Verification items for the finished model (mm, model axes). A direction names the side the tool comes from. Coordinates: 2 decimals unless noted, no trailing zeros. Write each loop counter-clockwise with the first axis right and the second up, starting at its lowest first coordinate (ties: lowest second). Pieces come first, ordered by that corner, then holes. Notation, with made-up numbers: (-5.5, 57.25) -> (45.5, 57.25) arc R33 ccw to (45.5, 87.25) -> close; hole circle Ø2 at (8.25, 37). An arc over 180 degrees is marked (long way). Answer in a Markdown table with one row per item.
```python
from build123d import *

# Parameters (mm, degrees)
F0_W      = 82.55
F0_H      = 38.1
F1_DEPTH  = 38.1
F2_W      = 57.15
F2_H      = 25.4
F3_DEPTH  = 38.101
F4_R      = 6.3636745149
F5_DEPTH  = 38.101
F7_DEPTH  = 25.4
F9_DEPTH  = 25.4
F10_DEPTH = 63.501
F12_DEPTH = 25.4


with BuildPart() as f1:
    # F0 (on Front) → F1 (new body)
    with BuildSketch(Plane.XZ):
        with Locations((-41.275, 19.05)):
            Rectangle(F0_W, F0_H)
    extrude(amount=F1_DEPTH)

    # F2 (on face) → F3 (cut, through all)
    with BuildSketch(Plane.XZ.offset(38.1)):
        with Locations((-28.575, 25.4)):
            Rectangle(F2_W, F2_H)
    extrude(amount=-F3_DEPTH, mode=Mode.SUBTRACT)

    # F4 (on face) → F5 (cut, through all)
    with BuildSketch(Plane.XZ.offset(38.1)):
        with Locations((-69.85, 25.9895079914)):
            Circle(F4_R)
    extrude(amount=-F5_DEPTH, mode=Mode.SUBTRACT)

    # F6 (on face) → F7 (cut)
    with BuildSketch(Plane.XY.offset(12.7)):
        with BuildLine():
            ThreePointArc((-43.1306947993, -12.7), (-38.6405667387, -14.5598719395), (-36.7806947993, -19.05))
            ThreePointArc((-36.7806947993, -19.05), (-38.6405667387, -23.5401280605), (-43.1306947993, -25.4))
            Line((-43.1306947993, -25.4), (-17.7306947993, -25.4))
            ThreePointArc((-17.7306947993, -25.4), (-24.0806947993, -19.05), (-17.7306947993, -12.7))
            Line((-17.7306947993, -12.7), (-43.1306947993, -12.7))
        make_face()
        with BuildLine():
            ThreePointArc((-43.1306947993, -25.4), (-38.6405667387, -23.5401280605), (-36.7806947993, -19.05))
            ThreePointArc((-36.7806947993, -19.05), (-38.6405667387, -14.5598719395), (-43.1306947993, -12.7))
            ThreePointArc((-43.1306947993, -12.7), (-49.4806947993, -19.05), (-43.1306947993, -25.4))
        make_face()
        with BuildLine():
            ThreePointArc((-11.3806947993, -19.05), (-13.2405667387, -14.5598719395), (-17.7306947993, -12.7))
            ThreePointArc((-17.7306947993, -12.7), (-24.0806947993, -19.05), (-17.7306947993, -25.4))
            ThreePointArc((-17.7306947993, -25.4), (-13.2405667387, -23.5401280605), (-11.3806947993, -19.05))
        make_face()
    extrude(amount=-F7_DEPTH, mode=Mode.SUBTRACT)

    # F8 (on face) → F9 (join)
    with BuildSketch(Plane.XZ.offset(38.1)):
        with BuildLine():
            ThreePointArc((-67.3090244137, 38.1), (-60.0909334069, 33.7845859546), (-57.15, 25.9058457722))
            Line((-57.15, 25.9058457722), (-57.15, 38.1))
            Line((-57.15, 38.1), (-67.3090244137, 38.1))
        make_face()
        with BuildLine():
            ThreePointArc((-82.55, 26.0334052145), (-79.5712875843, 33.8335010618), (-72.3941565633, 38.1))
            Line((-72.3941565633, 38.1), (-82.55, 38.1))
            Line((-82.55, 38.1), (-82.55, 26.0334052145))
        make_face()
    extrude(amount=F9_DEPTH)

    # F10 (cut, through all): faces of the model
    f10_faces = [f1.faces().sort_by_distance(p)[0] for p in [
        (-59.7492259595, -63.5, 35.2812720031),
        (-79.9507979007, -63.5, 35.2852151474),
    ]]
    extrude(f10_faces, amount=-F10_DEPTH, mode=Mode.SUBTRACT)

    # F11 (on face) → F12 (cut)
    with BuildSketch(Plane.XY.offset(12.7)):
        with BuildLine():
            ThreePointArc((-18.9558640122, 0), (-6.26601343, -5.5476288842), (0, -17.8985628462))
            Line((0, -17.8985628462), (0, 0))
            Line((0, 0), (-18.9558640122, 0))
        make_face()
        with BuildLine():
            ThreePointArc((0, -23.0064517831), (-3.2034542821, -31.7030229504), (-9.9095078185, -38.1))
            Line((-9.9095078185, -38.1), (0, -38.1))
            Line((0, -38.1), (0, -23.0064517831))
        make_face()
    extrude(amount=-F12_DEPTH, mode=Mode.SUBTRACT)


solid = f1.part
```
1. Section check C-C, the plane z = 7. Record the boundary of the cut face in (x, y), plus the area to 3 significant figures.
Geometry says:
| item | result |
|---|---|
| outline | (-82.55, -38.1) -> (-9.91, -38.1) arc R20.5 ccw to (0, -23.01) -> (0, -17.9) arc R20.5 ccw to (-18.96, 0) -> (-82.55, 0) -> close; hole (-43.13, -25.4) -> (-17.73, -25.4) arc R6.35 ccw to (-17.73, -12.7) -> (-43.13, -12.7) arc R6.35 ccw to start |
| area | 2,560 mm^2 |
2. Section check D-D, the plane y = -4.5. Record the boundary of the cut face in (x, z).
Geometry says:
| item | result |
|---|---|
| outline | (-82.55, 0) -> (-7.47, 0) -> (-7.47, 12.7) -> (-57.15, 12.7) -> (-57.15, 25.91) arc R12.7 ccw to (-67.31, 38.1) -> (-72.39, 38.1) arc R12.7 ccw to (-82.55, 26.03) -> close; hole circle Ø12.73 at (-69.85, 25.99) |
3. Tool access check on faces 4 (the flat face through (-30, -12.7, 6)), 5 (the cylindrical face through (-3.13, -31.59, 6.44)), 6 (the flat face through (-29, -28, 12.7)). Record the directions out of +Z, -Z, +X, -X, +Y, -Y that give a thin tool (end or side, any length) a straight path to the whole face; none if there is none.
Geometry says:
| item | result |
|---|---|
| face 4 | +Z, -Z |
| face 5 | +Z, -Z, +X, -Y |
| face 6 | +Z, +X, +Y, -Y |
4. Section check B-B, the plane x = -69.85. Record the boundary of the cut face in (y, z), plus the area to 3 significant figures.
Geometry says:
| item | result |
|---|---|
| outline | (-38.1, 0) -> (0, 0) -> (0, 19.63) -> (-38.1, 19.63) -> close; (-38.1, 32.35) -> (0, 32.35) -> (0, 38.1) -> (-38.1, 38.1) -> close |
| area | 967 mm^2 |
5. Mould release check, pull along Y, two halves, no side actions. Record for faces 1 (the cylindrical face through (-60.17, -19.32, 33.88)), 2 (the cylindrical face through (-49.48, -18.91, 6.44)), 3 (the flat face through (-58, 0, 15)): released by +Y, released by -Y, zero draft, split by the parting line, or undercut.
Geometry says:
| item | result |
|---|---|
| face 1 | zero draft |
| face 2 | undercut |
| face 3 | released by +Y |
6. Section check A-A, the plane y = -24. Record the boundary of the cut face in (x, z).
Geometry says:
| item | result |
|---|---|
| outline | (-82.55, 0) -> (-47.11, 0) -> (-47.11, 12.7) -> (-57.15, 12.7) -> (-57.15, 25.91) arc R12.7 ccw to (-67.31, 38.1) -> (-72.39, 38.1) arc R12.7 ccw to (-82.55, 26.03) -> close; (-13.75, 0) -> (-0.15, 0) -> (-0.15, 12.7) -> (-13.75, 12.7) -> close; hole circle Ø12.73 at (-69.85, 25.99) |
7. Depth check by flat-ended pin: P1, Ø6, axis at x = -20.5, y = -23.5, coming from the +Z side; P2, Ø10.5, axis at y = -14, z = 19.5, coming from the +X side. Enter the tip coordinate at first touch or a pass-through.
Geometry says:
| item | result |
|---|---|
| P1 | z = 12.7 |
| P2 | x = -57.15 |
8. Thickness scan on line 1 (Y direction, x = -23.5, z = 12); line 2 (Z direction, x = -69.85, y = -21); line 3 (Z direction, x = -8, y = -10.5). Record the ranges inside material, lowest first. Write a range as from..to.
Geometry says:
| item | result |
|---|---|
| line 1 | -38.1..-25.4, -12.7..0 |
| line 2 | 0..19.63, 32.35..38.1 |
| line 3 | 0..12.7 |
